The listing builds one solid part. Answer for the finished solid, in the listing's coordinates (mm). Face numbers are marked on the shaded views. A direction names the side the tool comes from. Give positions to 0.01 mm unless a question says otherwise; leave off trailing zeros. Write each loop counter-clockwise with the first axis right and the second up, starting at its lowest first coordinate (ties: lowest second). Pieces come first, ordered by that corner, then holes. Notation, with made-up numbers: (65.25, 80) - (95.25, 80) arc R16 cw to (95.25, 109) - close; hole circle Ø7 at (84, 83.5). An arc over 180 degrees is marked (long way). Answer as CSV lines item,"result". Start each with the question number.
(1) For the marked faces 4, 5 and 6, determine the directions among +Z, -Z, +X, -X, +Y, -Y from which every point of the face is accessible in a straight line to the end or side of a thin tool.
(2) Find section A-A (x = 20). Write down the section's boundary in (y, z), then the cut area to 3 significant figures.
(3) Find section D-D (y = -4.75). State how many separate pieces and enclosed holes the cut face has, then the cut area to 3 significant figures.
(4) Straight lines are drawn through the part: probe 1 along X at (y, z) = (-2, 5); probe 2 along X at (y, z) = (-0.25, 12); probe 3 along Z at (x, y) = (36.5, -3.5). For each, find the intervals that lie inside material, in ascending order.
(5) For a pull along Z with two mould halves and no side action, classify the marked faces 1, 2 and 3 as pulls with the +Z half, pulls with the -Z half, needs draft (parallel to the pull), parting line crosses it, or undercut.
(6) Find section B-B (z = 42.5). Write down the section's boundary in (x, y), then the cut area to 3 significant figures.
(7) Each of these flat-tipped pins is pushed along its axis until it touches: pin 1 Ø1.5 at (y, z) = (-1, 38) entering from -X; pin 2 Ø2 at (x, y) = (22, -2) entering from -Z; pin 3 Ø1.5 at (x, y) = (48, -3.5) entering from +Z. Where does it stop, or does it pass through?
(8) Find section C-C (z = 14). Write down the section's boundary in (x, y).
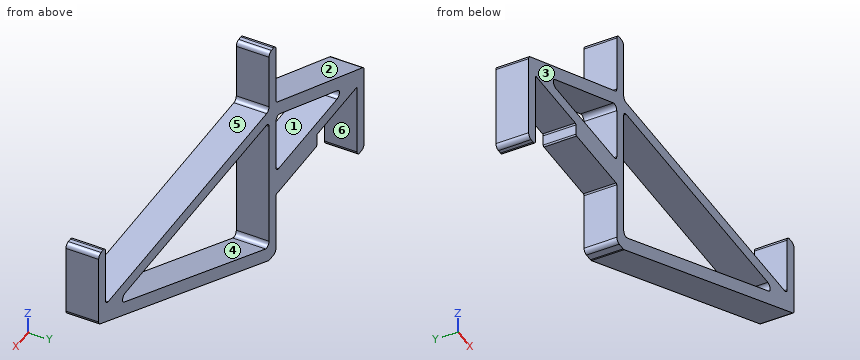
from build123d import *

# Parameters (mm, degrees)
F0_W     = 14.9098
F0_H     = 2.54
F0_W_2   = 2.54
F0_H_2   = 12.7
F1_DEPTH = 6.35
F2_R     = 0.889
F3_R     = 0.254


# Not quite as in the source:
# - a feature names something its author has since deleted; it is built from what else it names


with BuildPart() as f1:
    # F0 (on Front) → F1 (new body)
    with BuildSketch(Plane.XZ):
        Polygon((32.1818, 20.32), (32.1818, 17.78), (34.7218, 17.78), (34.7218, 30.48), (34.7218, 33.02), (32.1818, 33.02), (32.1818, 30.2095859146), align=None)
        Polygon((34.7218, 17.78), (32.1818, 17.78), (32.1818, 15.24), (32.1818, 12.7), (32.1818, 0), (34.7218, 0), (34.7218, 2.8283102922), (34.7218, 13.97), align=None)
        Polygon((0, 17.78), (2.54, 17.78), (5.9346577437, 17.78), (32.1818, 30.2095859146), (32.1818, 33.02), align=None)
        Polygon((5.9346577437, 17.78), (2.54, 17.78), (2.54, 15.24), (17.272, 15.24), (32.1818, 15.24), (32.1818, 17.78), align=None)
        with Locations((24.7269, 13.97)):
            Rectangle(F0_W, F0_H)
        Polygon((2.54, 15.24), (2.54, 17.78), (0, 17.78), (0, 0), (2.54, 0), align=None)
        Polygon((91.1773331535, 30.48), (34.7218, 2.8283102922), (34.7218, 0), (96.9518, 30.48), align=None)
        Polygon((94.4118, 33.02), (34.7218, 33.02), (34.7218, 30.48), (91.1773331535, 30.48), (96.9518, 30.48), (96.9518, 33.02), align=None)
        with Locations((95.6818, 39.37)):
            Rectangle(F0_W_2, F0_H_2)
        with Locations((33.4518, 39.37)):
            Rectangle(F0_W_2, F0_H_2)
    extrude(amount=F1_DEPTH)

    # F2
    f2_edges = [f1.edges().sort_by_distance(p)[0] for p in [
        (0, -3.175, 0),
        (2.54, -3.175, 0),
        (32.1818, -3.175, 0),
        (34.7218, -3.175, 0),
        (32.1818, -3.175, 33.02),
        (0, -3.175, 17.78),
        (32.1818, -3.175, 17.78),
        (32.1818, -3.175, 30.209586),
        (5.934658, -3.175, 17.78),
        (34.7218, -3.175, 2.82831),
        (34.7218, -3.175, 30.48),
        (91.177333, -3.175, 30.48),
        (96.9518, -3.175, 30.48),
        (96.9518, -3.175, 45.72),
        (94.4118, -3.175, 45.72),
        (94.4118, -3.175, 33.02),
        (32.1818, -3.175, 45.72),
        (34.7218, -3.175, 45.72),
        (34.7218, -3.175, 33.02),
    ]]
    fillet(f2_edges, radius=F2_R)

    # F3
    f3_edges = [f1.edges().sort_by_distance(p)[0] for p in [
        (2.54, -3.175, 15.24),
        (17.272, -3.175, 15.24),
        (17.272, -3.175, 12.7),
        (32.1818, -3.175, 12.7),
    ]]
    fillet(f3_edges, radius=F3_R)


solid = f1.part
Result set:
1,face 4,"+Y, -Y"
1,face 5,"+Z, +Y, -Y"
1,face 6,"-Z, +Y, -Y"
2,outline,"(-6.35, 12.7) - (0, 12.7) - (0, 17.78) - (-6.35, 17.78) - close; (-6.35, 24.44) - (0, 24.44) - (0, 27.25) - (-6.35, 27.25) - close"
2,area,"50.1 mm^2"
3,separate pieces,"1"
3,enclosed holes,"2"
3,area,"720 mm^2"
4,probe 1,"0 to 2.54, 32.18 to 34.72, 39.16 to 44.93"
4,probe 2,"0 to 2.54, 32.18 to 34.72, 53.45 to 59.22"
4,probe 3,"0.87 to 3.7, 30.48 to 33.02"
5,face 1,"undercut"
5,face 2,"pulls with the +Z half"
5,face 3,"needs draft"
6,outline,"(32.18, -6.35) - (34.72, -6.35) - (34.72, 0) - (32.18, 0) - close; (94.41, -6.35) - (96.95, -6.35) - (96.95, 0) - (94.41, 0) - close"
6,area,"32.3 mm^2"
7,pin 1,"x = 32.18"
7,pin 2,"z = 12.7"
7,pin 3,"z = 33.02"
8,outline,"(0, -6.35) - (2.54, -6.35) - (2.54, 0) - (0, 0) - close; (17.27, -6.35) - (34.72, -6.35) - (34.72, 0) - (17.27, 0) - close; (57.53, -6.35) - (63.31, -6.35) - (63.31, 0) - (57.53, 0) - close"
